from build123d import *

# Parameters (mm, degrees)
ESQUISSE1_R        = 2
BOSS_EXTRU_1_DEPTH = 45
CONG_1_R           = 0.75


with BuildPart() as part:
    # Esquisse1 → Boss.-Extru.1 (new body)
    with BuildSketch(Plane(origin=(0, 0, 0), x_dir=(0, 0, -1), z_dir=(1, 0, 0))):
        Polygon((2.5, 10), (10, 10), (10, 2.5), (8.5, 2.5), (8.5, 7.439339828), (3.75, 2.689339828), (3.75, -2.689339828), (8.5, -7.439339828), (8.5, -2.5), (10, -2.5), (10, -10), (2.5, -10), (2.5, -8.5), (7.439339828, -8.5), (2.689339828, -3.75), (-2.689339828, -3.75), (-7.439339828, -8.5), (-2.5, -8.5), (-2.5, -10), (-10, -10), (-10, -2.5), (-8.5, -2.5), (-8.5, -7.439339828), (-3.75, -2.689339828), (-3.75, 2.689339828), (-8.5, 7.439339828), (-8.5, 2.5), (-10, 2.5), (-10, 10), (-2.5, 10), (-2.5, 8.5), (-7.439339828, 8.5), (-2.689339828, 3.75), (2.689339828, 3.75), (7.439339828, 8.5), (2.5, 8.5), align=None)
        with Locations(Location((0, 0, 0), (0, 0, 180))):
            Circle(ESQUISSE1_R, mode=Mode.SUBTRACT)
    extrude(amount=BOSS_EXTRU_1_DEPTH)

    # Congé1
    cong_1_edges = [part.edges().sort_by_distance(p)[0] for p in [
        (22.5, 7.439339828, -8.5),
        (22.5, -7.439339828, -8.5),
        (22.5, -8.5, -7.439339828),
        (22.5, -8.5, 7.439339828),
        (22.5, -7.439339828, 8.5),
        (22.5, 7.439339828, 8.5),
        (22.5, 8.5, 7.439339828),
        (22.5, 8.5, -7.439339828),
    ]]
    fillet(cong_1_edges, radius=CONG_1_R)


solid = part.part
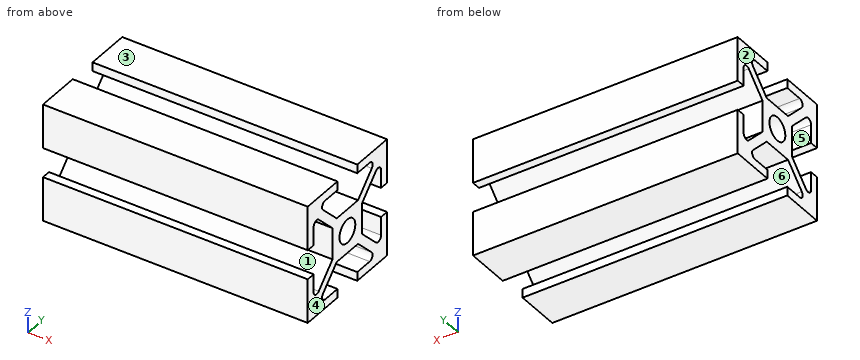
Build history of the part. All positions in model axes, mm. Face numbers are marked on the shaded views. A direction names the side the tool comes from. Coordinates: 2 decimals unless noted, no trailing zeros. Write each loop counter-clockwise with the first axis right and the second up, starting at its lowest first coordinate (ties: lowest second). Pieces come first, ordered by that corner, then holes.
(1) Drill centre lines: line 1 (Y direction, x = 26.5, z = 0); line 2 (Y direction, x = 25, z = 5.75); line 3 (Z direction, x = 4.5, y = 2.75). Where is each one in solid material? Low to high.
(2) Cut at C-C on z = -5. List the corners of the cut face in (x, y).
(3) Cut at A-A on y = 0. List the corners of the cut face in (x, z).
(4) Pin check, flat tips, straight feed: pin 1 Ø2.5 at (x, y) = (32, 0.5) entering from -Z; pin 2 Ø1.6 at (x, z) = (18.5, 0) entering from -Y. Stop position of each tip, or through.
(5) Mould opens along Z. For the marked faces 3, 4, 5 and 6 say: pulls with the +Z half, pulls with the -Z half, needs draft (parallel to the pull), parting line crosses it, or undercut.
(6) 3-axis set-ups, long thin cutter, end or side, ignore diameter. For the marked faces 1 and 2: which of +Z, -Z, +X, -X, +Y, -Y reach the whole face in a straight line?
Working result:
1. line 1: y = -3.75 to -2, 2 to 3.75
1. line 2: y = -10 to -8.49, -6.81 to -4.69, 4.69 to 6.81, 8.49 to 10
1. line 3: z = -10 to -8.5, -3.81 to 3.81, 8.5 to 10
2. outline: (0, -10) - (45, -10) - (45, -8.5) - (0, -8.5) - close; (0, -6.06) - (45, -6.06) - (45, -3.94) - (0, -3.94) - close; (0, 3.94) - (45, 3.94) - (45, 6.06) - (0, 6.06) - close; (0, 8.5) - (45, 8.5) - (45, 10) - (0, 10) - close
3. outline: (0, -3.75) - (45, -3.75) - (45, -2) - (0, -2) - close; (0, 2) - (45, 2) - (45, 3.75) - (0, 3.75) - close
4. pin 1: stops at z = -3.75
4. pin 2: stops at y = -3.75
5. face 3: pulls with the +Z half
5. face 4: needs draft
5. face 5: undercut
5. face 6: undercut
6. face 1: +X, -X
6. face 2: +Z, -Z, -X, +Y, -Y
